Here's how the part is built. I have some questions about the finished solid (model axes, mm). A direction names the side the tool comes from. Round coordinates to 2 decimals unless told otherwise and drop trailing zeros. Order: outer loops, then holes, each group sorted by start corner. A loop starts at its lowest first (then second) coordinate and runs counter-clockwise, first axis right, second up.
```python
from build123d import *

# Parameters (mm, degrees)
BOSS_EXTRUDE1_DEPTH = 45.3
SKETCH2_R           = 1.65
CUT_EXTRUDE1_DEPTH  = 50.873239317
SKETCH3_R           = 1.5
CUT_EXTRUDE2_DEPTH  = 51.797047158


with BuildPart() as part:
    # Sketch1 → Boss-Extrude1 (new body)
    with BuildSketch(Plane.XY):
        Polygon((0, 0), (0, 18), (-1.5, 18), (-1.5, 1.5), (-16, 1.5), (-16, 0), align=None)
    extrude(amount=BOSS_EXTRUDE1_DEPTH)

    # Sketch2 → Cut-Extrude1 (cut, through all)
    with BuildSketch(Plane(origin=(-1.5, 3, 0), x_dir=(0, 1, 0), z_dir=(-1, 0, 0))):
        Polygon((12, 0), (15, -3), (15, 0), align=None)
        Polygon((15, -42.3), (12, -45.3), (15, -45.3), align=None)
        with Locations(Location((6, -14.3, 0), (0, 0, 270))):
            Circle(SKETCH2_R)
        with Locations(Location((6, -31, 0), (0, 0, 90))):
            Circle(SKETCH2_R)
    extrude(amount=-CUT_EXTRUDE1_DEPTH, mode=Mode.SUBTRACT)

    # Sketch3 → Cut-Extrude2 (cut, through all)
    with BuildSketch(Plane(origin=(0, 1.5, 0), x_dir=(1, 0, 0), z_dir=(0, 1, 0))):
        with Locations(Location((-7.5, -4.15, 0), (0, 0, 270))):
            Circle(SKETCH3_R)
        with Locations(Location((-7.5, -41.15, 0), (0, 0, 90))):
            Circle(SKETCH3_R)
    extrude(amount=-CUT_EXTRUDE2_DEPTH, mode=Mode.SUBTRACT)


solid = part.part
```
1) If we section it at C-C (y = 9): Write out the boundary of the cut face in (x, z), plus the area to 4 significant figures.
2) If we section it at D-D (z = 31): Write out the boundary of the cut face in (x, y), plus the area to 3 significant figures.
3) We'd pull the mould along X, two halves only. Please class faces 1 (the cylindrical face through (-0.76, 8.93, 32.65)), 2 (the cylindrical face through (-8.964, 0.76, 3.825)), 3 (the flat face through (-16, 1, 22)): +X half, -X half, draft (parallel to the pull), parting line (faces both ways), or undercut.
4) I need wall thicknesses on line 1 (Y direction, x = -0.85, z = 31); line 2 (X direction, y = 0.8, z = 4.15); line 3 (X direction, y = 17, z = 28). Which ranges of each line are inside material? Lowest first, please.
5) For faces 4 (the flat face through (-1, 16, 1)), 5 (the flat face through (-9, 1.5, 22)), which set-ups out of +Z, -Z, +X, -X, +Y, -Y let a thin tool reach every point of the face, with its end or its side?
6) I'm going to push flat-ended pins straight in: pin 1 (2 mm diameter, centred on x = -5.5, z = 21.5, fed in from +Y); pin 2 (8 mm diameter, centred on y = 6, z = 29, fed in from -X). Where does each tip first touch, or does it pass through?
7) If we section it at B-B (x = -7.5): Write out the boundary of the cut face in (y, z).
8) If we section it at A-A (z = 41.15): Write out the boundary of the cut face in (x, y).
Solutions:
1. outline: (-1.5, 0) - (0, 0) - (0, 12.65) - (-1.5, 12.65) - close; (-1.5, 15.95) - (0, 15.95) - (0, 29.35) - (-1.5, 29.35) - close; (-1.5, 32.65) - (0, 32.65) - (0, 45.3) - (-1.5, 45.3) - close
1. area: 58.05 mm2
2. outline: (-16, 0) - (0, 0) - (0, 7.35) - (-1.5, 7.35) - (-1.5, 1.5) - (-16, 1.5) - close; (-1.5, 10.65) - (0, 10.65) - (0, 18) - (-1.5, 18) - close
2. area: 43.8 mm2
3. face 1: draft
3. face 2: undercut
3. face 3: -X half
4. line 1: y = 0 to 7.35, 10.65 to 18
4. line 2: x = -16 to -9, -6 to 0
4. line 3: x = -1.5 to 0
5. face 4: -Z, +X, -X, +Y
5. face 5: +Z, -Z, -X, +Y
6. pin 1: stops at y = 1.5
6. pin 2: stops at x = -1.5
7. outline: (0, 0) - (1.5, 0) - (1.5, 2.65) - (0, 2.65) - close; (0, 5.65) - (1.5, 5.65) - (1.5, 39.65) - (0, 39.65) - close; (0, 42.65) - (1.5, 42.65) - (1.5, 45.3) - (0, 45.3) - close
8. outline: (-16, 0) - (-9, 0) - (-9, 1.5) - (-16, 1.5) - close; (-6, 0) - (0, 0) - (0, 18) - (-1.5, 18) - (-1.5, 1.5) - (-6, 1.5) - close
